Build history of the part. All positions in model axes, mm. Give positions to 0.01 mm unless a question says otherwise; leave off trailing zeros. Loops run counter-clockwise (first coordinate to the right, second up) from the corner with the lowest first, then second, coordinate; pieces in that order, holes last. Notation, with made-up numbers: M 9,14.25 L 50,14.25 A13 cw 50,20.25 Z; hole C 25,-32.5 d7. An arc over 180 degrees is marked long. Answer as a JSON object with one key per item and string values. Group by question number.
1. Drop flat-ended pins along their axis: pin 1 Ø2 at (x, y) = (-8, 8.75) entering from +Z; pin 2 Ø1.5 at (y, z) = (-3, 2.5) entering from +X; pin 3 Ø1.2 at (x, y) = (5.5, 8.75) entering from -Z; pin 4 Ø0.8 at (x, z) = (0, 2.5) entering from -Y. Give the stop position or say it passes through.
2. Slice it at D-D (x = 4.5). List the corners of the cut face in (y, z).
3. Drill centre lines: line 1 along Y through (x, z) = (8, 0.3); line 2 along Y through (x, z) = (-3, 0.3); line 3 along Z through (x, y) = (4, -7.5). Where is each one in solid material? Low to high. Write a range as [from, to].
4. Slice it at A-A (x = -5.5). List the corners of the cut face in (y, z), then the cut area to 3 significant figures.
5. Slice it at B-B (y = -8.75). List the corners of the cut face in (x, z), then the cut area to 3 significant figures.
6. Slice it at C-C (z = 1). Give the number of separate pieces and of enclosed holes in the cut face, then the cut area to 3 significant figures.
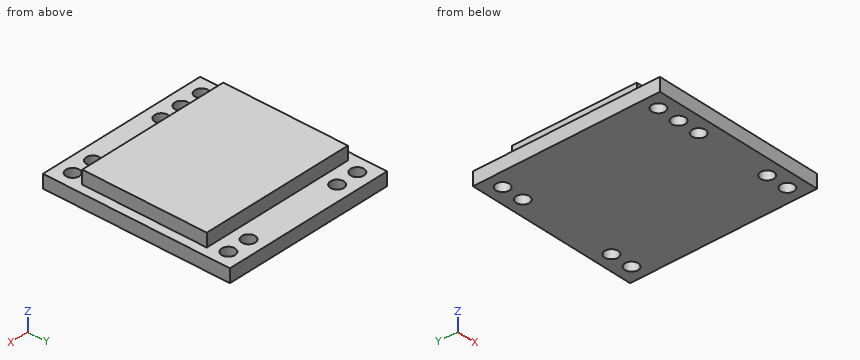
from build123d import *

# Parameters (mm, degrees)
F0_W     = 19.5
F0_H     = 21
F0_R     = 0.75
F0_W_2   = 17.5
F0_H_2   = 14
F1_DEPTH = 1.5
F2_DEPTH = 3


with BuildPart() as f1:
    # F0 (on Top) → F1 (new body)
    with BuildSketch(Plane.XY):
        Rectangle(F0_W, F0_H)
        with Locations((-8, -8.75)):
            Circle(F0_R, mode=Mode.SUBTRACT)
        with Locations((-5.5, -8.75)):
            Circle(F0_R, mode=Mode.SUBTRACT)
        with Locations((-3, -8.75)):
            Circle(F0_R, mode=Mode.SUBTRACT)
        with Locations((5.5, -8.75)):
            Circle(F0_R, mode=Mode.SUBTRACT)
        with Locations((8, -8.75)):
            Circle(F0_R, mode=Mode.SUBTRACT)
        with Locations((-8, 8.75)):
            Circle(F0_R, mode=Mode.SUBTRACT)
        with Locations((-5.5, 8.75)):
            Circle(F0_R, mode=Mode.SUBTRACT)
        Rectangle(F0_W_2, F0_H_2, mode=Mode.SUBTRACT)
        with Locations((5.5, 8.75)):
            Circle(F0_R, mode=Mode.SUBTRACT)
        with Locations((8, 8.75)):
            Circle(F0_R, mode=Mode.SUBTRACT)
    extrude(amount=F1_DEPTH)

    # F0 (on Top) → F2 (join)
    with BuildSketch(Plane.XY):
        Rectangle(F0_W_2, F0_H_2)
    extrude(amount=F2_DEPTH)


solid = f1.part
Established:
{
 "1": {"pin 1": "stops at z = 1.5", "pin 2": "stops at x = 8.75", "pin 3": "passes through", "pin 4": "stops at y = -7"},
 "2": {"outline": "M -10.5,0 L 10.5,0 L 10.5,1.5 L 7,1.5 L 7,3 L -7,3 L -7,1.5 L -10.5,1.5 Z"},
 "3": {"line 1": "y = [-10.5, -9.5], [-8, 8], [9.5, 10.5]", "line 2": "y = [-10.5, -9.5], [-8, 10.5]", "line 3": "z = [0, 1.5]"},
 "4": {"outline": "M -10.5,0 L -9.5,0 L -9.5,1.5 L -10.5,1.5 Z; M -8,0 L 8,0 L 8,1.5 L 7,1.5 L 7,3 L -7,3 L -7,1.5 L -8,1.5 Z; M 9.5,0 L 10.5,0 L 10.5,1.5 L 9.5,1.5 Z", "area": "48.0 mm^2"},
 "5": {"outline": "M -9.75,0 L -8.75,0 L -8.75,1.5 L -9.75,1.5 Z; M -7.25,0 L -6.25,0 L -6.25,1.5 L -7.25,1.5 Z; M -4.75,0 L -3.75,0 L -3.75,1.5 L -4.75,1.5 Z; M -2.25,0 L 4.75,0 L 4.75,1.5 L -2.25,1.5 Z; M 6.25,0 L 7.25,0 L 7.25,1.5 L 6.25,1.5 Z; M 8.75,0 L 9.75,0 L 9.75,1.5 L 8.75,1.5 Z", "area": "18.0 mm^2"},
 "6": {"separate pieces": "1", "enclosed holes": "9", "area": "394 mm^2"}
}
